Can you work these out from the model? Positions are in its coordinate system, mm. A direction names the side the tool comes from. Round coordinates to 2 decimals unless told otherwise and drop trailing zeros. Order: outer loops, then holes, each group sorted by start corner. A loop starts at its lowest first (then second) coordinate and runs counter-clockwise, first axis right, second up. Notation, with made-up numbers: M -30.75,37 L 6.25,37 A13 cw 6.25,57 Z; hole C 49.25,18.5 d4. An arc over 180 degrees is marked long. Answer as a JSON object with one key per item and string values. Group by question number.
```python
from build123d import *

# Parameters (mm, degrees)
SKETCH_1_R          = 2.5
EXTRUDE_1_DEPTH     = 5
SKETCH_2_W          = 50
SKETCH_2_H          = 50
EXTRUDE_2_DEPTH     = 11.5
SKETCH_3_R          = 11.5
CUT_EXTRUDE_1_DEPTH = 203.131763956
SKETCH_1_7_R        = 2.5
CUT_EXTRUDE_3_DEPTH = 251.264360227


with BuildPart() as part:
    # Sketch 1 → Extrude 1 (new body)
    with BuildSketch(Plane(origin=(0, 0, 0), x_dir=(1, 0, 0), z_dir=(0, 1, 0))):
        with BuildLine():
            Line((0, 0), (-180, 0))
            ThreePointArc((-180, 0), (-194.142135624, 5.857864376), (-200, 20))
            Line((-200, 20), (-200, 130))
            ThreePointArc((-200, 130), (-194.142135624, 144.142135624), (-180, 150))
            Line((-180, 150), (-108.660254038, 150))
            ThreePointArc((-108.660254038, 150), (-103.483873136, 149.318516526), (-98.660254038, 147.320508076))
            Line((-98.660254038, 147.320508076), (-70, 130.773502692))
            ThreePointArc((-70, 130.773502692), (-62.679491924, 123.452994616), (-60, 113.452994616))
            Line((-60, 113.452994616), (-60, 65))
            ThreePointArc((-60, 65), (-54.142135624, 50.857864376), (-40, 45))
            Line((-40, 45), (0, 45))
            Line((0, 45), (0, 0))
        make_face()
        with Locations(Location((-127.5, 57.5, 0), (0, 0, 270))):
            Circle(SKETCH_1_R, mode=Mode.SUBTRACT)
        with Locations(Location((-92.5, 57.5, 0), (0, 0, 270))):
            Circle(SKETCH_1_R, mode=Mode.SUBTRACT)
        with Locations(Location((-127.5, 22.5, 0), (0, 0, 270))):
            Circle(SKETCH_1_R, mode=Mode.SUBTRACT)
        with Locations(Location((-92.5, 22.5, 0), (0, 0, 270))):
            Circle(SKETCH_1_R, mode=Mode.SUBTRACT)
        with Locations(Location((-170, 110, 0), (0, 0, 270))):
            Circle(SKETCH_1_R, mode=Mode.SUBTRACT)
        with Locations(Location((-90, 110, 0), (0, 0, 270))):
            Circle(SKETCH_1_R, mode=Mode.SUBTRACT)
        with Locations(Location((-170, 30, 0), (0, 0, 270))):
            Circle(SKETCH_1_R, mode=Mode.SUBTRACT)
    extrude_1 = extrude(amount=EXTRUDE_1_DEPTH)

    # Sketch 2 → Extrude 2 (add)
    with BuildSketch(Plane(origin=(0, 0, 0), x_dir=(1, 0, 0), z_dir=(0, 1, 0))):
        with Locations((-110, 40)):
            Rectangle(SKETCH_2_W, SKETCH_2_H)
    extrude_2 = extrude(amount=-EXTRUDE_2_DEPTH)

    # Sketch 3 → Cut-Extrude 1 (cut, through all)
    with BuildSketch(Plane.ZY.offset(135)):
        with Locations((-40, -11.5)):
            Circle(SKETCH_3_R)
    cut_extrude_1 = extrude(amount=-CUT_EXTRUDE_1_DEPTH, mode=Mode.SUBTRACT)

    # Sketch 1_7 → Cut-Extrude 3 (cut, through all)
    with BuildSketch(Plane(origin=(0, 0, 0), x_dir=(1, 0, 0), z_dir=(0, 1, 0))):
        with Locations(Location((-127.5, 57.5, 0), (0, 0, 270))):
            Circle(SKETCH_1_7_R)
        with Locations(Location((-92.5, 57.5, 0), (0, 0, 270))):
            Circle(SKETCH_1_7_R)
        with Locations(Location((-127.5, 22.5, 0), (0, 0, 270))):
            Circle(SKETCH_1_7_R)
        with Locations(Location((-92.5, 22.5, 0), (0, 0, 270))):
            Circle(SKETCH_1_7_R)
    cut_extrude_3 = extrude(amount=-CUT_EXTRUDE_3_DEPTH, mode=Mode.SUBTRACT)

    # Mirror 1: Extrude 1, Extrude 2, Cut-Extrude 1, Cut-Extrude 3 across plane
    add(extrude_1.mirror(Plane(origin=(0, 5, -45), x_dir=(0, 0, 1), z_dir=(-1, 0, 0))))
    add(extrude_2.mirror(Plane(origin=(0, 5, -45), x_dir=(0, 0, 1), z_dir=(-1, 0, 0))))
    add(cut_extrude_1.mirror(Plane(origin=(0, 5, -45), x_dir=(0, 0, 1), z_dir=(-1, 0, 0))), mode=Mode.SUBTRACT)
    add(cut_extrude_3.mirror(Plane(origin=(0, 5, -45), x_dir=(0, 0, 1), z_dir=(-1, 0, 0))), mode=Mode.SUBTRACT)


solid = part.part
```
1) I need wall thicknesses on line 1 along Z through (x, y) = (-170, 2.7); line 2 along X through (y, z) = (3.4, -30); line 3 along X through (y, z) = (-3, -18). Which ranges of each line are inside material? Lowest first, please.
2) If we section it at B-B on x = 19.5: Write out the boundary of the cut face in (y, z), plus the area to 3 significant figures.
3) For pin 1 (4.5 mm diameter, centred on x = -90, z = -110, fed in from -Y); pin 2 (5 mm diameter, centred on x = -26, y = -1, fed in from -Z); pin 3 (3.5 mm diameter, centred on x = -108, y = -3, fed in from -Z); pin 4 (6 mm diameter, centred on y = -6.5, z = -57, fed in from +X), each with a flat end and sliding along its axis, tell me the tip position at first contact or that it passes through.
4) We'd pull the mould along X, two halves only. Please class faces 1 (the face through (85, -6, -22)), 2 (the face through (194.297, 2.465, -143.986)), 3 (the face through (110, -11.5, -58)): +X half, -X half, draft (parallel to the pull), parting line (faces both ways), or undercut.
5) Which directions (+Z, -Z, +X, -X, +Y, -Y) give clear straight access to the entire face, cutting with the end or side of a thin tool? Please do faces 4 (the face through (54.297, 2.465, -51.014)), 5 (the face through (110, -6, -15)), 6 (the face through (135, -6, -58)), 7 (the face through (-85, -6, -22)).
6) If we section it at A-A on y = -7.25: Count the separate pieces of the cut face and the enclosed holes in it, plus the area to 3 significant figures.
7) If we section it at C-C on z = -11: Write out the boundary of the cut face in (x, y), plus the area to 3 significant figures.
Findings:
{
 "1": {"line 1": "z = -150 to -112.5, -107.5 to -32.5, -27.5 to 0", "line 2": "x = -200 to -172.5, -167.5 to 167.5, 172.5 to 200", "line 3": "x = -135 to -85, 85 to 135"},
 "2": {"outline": "M 0,-45 L 5,-45 L 5,0 L 0,0 Z", "area": "225 mm^2"},
 "3": {"pin 1": "passes through", "pin 2": "stops at z = -45", "pin 3": "stops at z = -65", "pin 4": "stops at x = 135"},
 "4": {"face 1": "undercut", "face 2": "+X half", "face 3": "draft"},
 "5": {"face 4": "-Z, +Y, -Y", "face 5": "+Z, +X, -X, -Y", "face 6": "+Z, -Z, +X, -Y", "face 7": "+Z, -Z, -Y"},
 "6": {"separate pieces": "4", "enclosed holes": "8", "area": "2,710 mm^2"},
 "7": {"outline": "M -197.86,0 L 197.86,0 L 197.86,5 L -197.86,5 Z", "area": "1,980 mm^2"}
}
